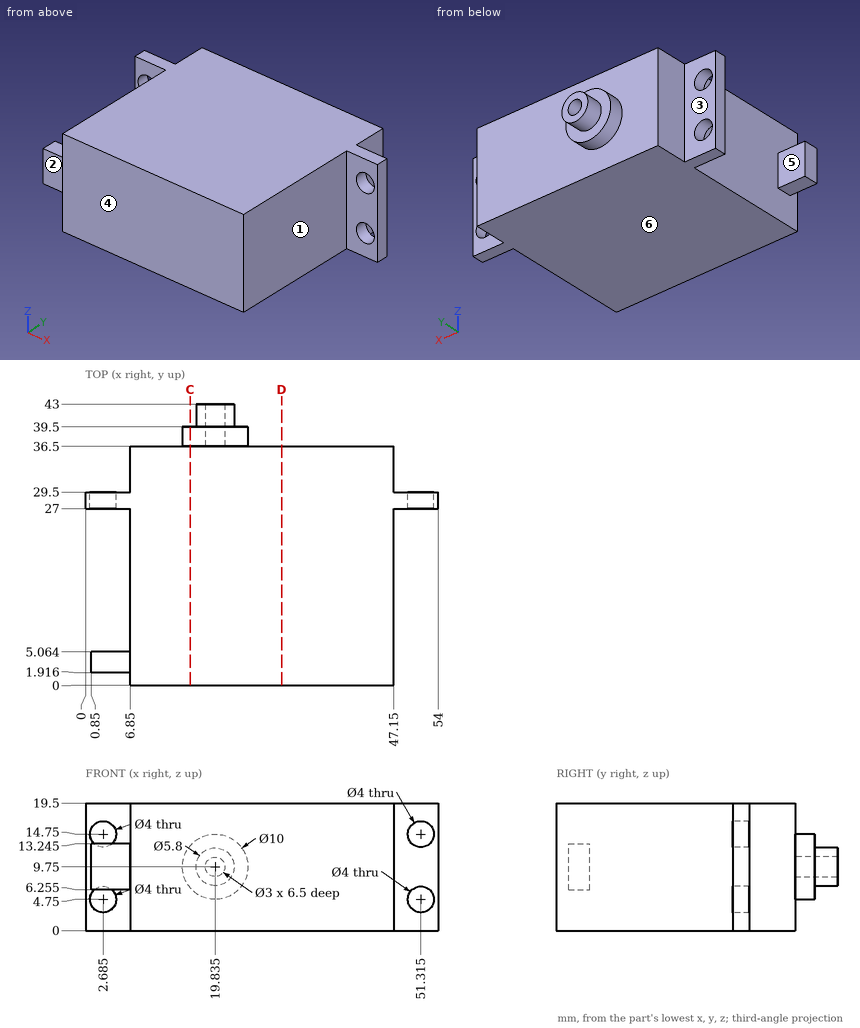
For this review, use the dimensioned drawing (mm, ordinates from the lowest corner) and the shaded views. A direction names the side the tool comes from. Round coordinates to 2 decimals unless told otherwise and drop trailing zeros. Write each loop counter-clockwise with the first axis right and the second up, starting at its lowest first coordinate (ties: lowest second). Pieces come first, ordered by that corner, then holes. Notation, with made-up numbers: (83, 50) -> (102, 50) arc R19 ccw to (102, 74) -> close; hole circle Ø1 at (30, -31.75). An arc over 180 degrees is marked (long way). Use CSV: the item, a comma, the result in double quotes.
Q1. Consider section D-D (x = 30). Give the boundary of the cut face in (y, z).
Checks:
outline,"(0, 0) -> (36.5, 0) -> (36.5, 19.5) -> (0, 19.5) -> close"
Q2. To check wall thickness, follow probe 1 along X at (y, z) = (27.85, 14.75) (1 decimal); probe 2 along Y at (x, z) = (5, 7) (1 decimal); probe 3 along X at (y, z) = (41.25, 9.75) (1 decimal). State the ranges of each line that lie inside material, in increasing order. Write a range as [from, to].
Checks:
probe 1,"[0, 0.7], [4.7, 49.3], [53.3, 54]"
probe 2,"[1.9, 5.1], [27, 29.5]"
probe 3,"[16.9, 18.3], [21.3, 22.7]"
Q3. Mouldability with a two-part tool opening along Y and no side actions: class the marked faces 4, 5 and 6 as released by +Y, released by -Y, zero draft, split by the parting line, or undercut.
Checks:
face 4,"released by -Y"
face 5,"undercut"
face 6,"zero draft"
Q4. For pin 1 Ø2 at (y, z) = (32.5, 8) entering from -X; pin 2 Ø6.5 at (x, z) = (2.5, 11) entering from -Y; pin 3 Ø0.9 at (y, z) = (4, 9) entering from -X; pin 4 Ø2.5 at (x, z) = (51.315, 14.75) entering from +Y, all flat-tipped, find the tip position at first contact; note any pin that passes through.
Checks:
pin 1,"x = 6.85"
pin 2,"y = 1.92"
pin 3,"x = 0.85"
pin 4,"through"
Q5. For the marked faces 1, 2 and 3, list the 3-axis set-ups (+Z, -Z, +X, -X, +Y, -Y) from which the entire face can be reached by the end or side of a thin tool; tool diameter is ignored.
Checks:
face 1,"+Z, -Z, +X, -Y"
face 2,"+Z, -Z, -X, -Y"
face 3,"+Z, -Z, -X, +Y"
Q6. Consider section C-C (x = 16). Give the boundary of the cut face in (y, z).
Checks:
outline,"(0, 0) -> (36.5, 0) -> (36.5, 6.54) -> (39.5, 6.54) -> (39.5, 12.96) -> (36.5, 12.96) -> (36.5, 19.5) -> (0, 19.5) -> close"
